The listing builds one solid part. Answer for the finished solid, in the listing's coordinates (mm). Face numbers are marked on the shaded views. Round coordinates to 2 decimals unless told otherwise and drop trailing zeros. Order: outer loops, then holes, each group sorted by start corner. A loop starts at its lowest first (then second) coordinate and runs counter-clockwise, first axis right, second up. Notation, with made-up numbers: (-22.5, 52) -> (-1.5, 52) arc R22 ccw to (-1.5, 78) -> close; hole circle Ø10 at (-11, 1). An arc over 180 degrees is marked (long way). Return JSON: item names as keys, results as strings. Group by question number.
(1) Consider line 1 (Y direction, x = 0, z = 4.4) (3 decimals); line 2 (X direction, y = 0.75, z = 3.7); line 3 (X direction, y = 0.25, z = 0.9). Determine where each line is inside the solid, lowest interval first. Write a range as [from, to].
(2) The part is cut by section D-D (y = 5.75). Determine the outline of the cut face in (x, z).
(3) Determine the mould class of the marked faces 1, 2 and 3 for opening direction Y: +Y half, -Y half, draft (parallel to the pull), parting line (faces both ways), or undercut.
(4) The part is cut by section A-A (z = 3.8). Determine the outline of the cut face in (x, y) (3 decimals).
(5) Each of these flat-tipped pins is pushed along its axis until it touches: pin 1 (2 mm diameter, centred on y = 2.5, z = 3.5, fed in from -X); pin 2 (1 mm diameter, centred on x = -3.5, z = 2.5, fed in from -Y). Where does it stop, or does it pass through?
(6) The part is cut by section C-C (x = -3.25). Determine the outline of the cut face in (y, z), plus the area to 3 significant figures.
(7) The part is cut by section B-B (y = -1). Determine the outline of the cut face in (x, z).
from build123d import *

# Parameters (mm, degrees)
F1_DEPTH = 6


# Not quite as in the source:
# - a feature names something its author has since deleted; it is built from what else it names


with BuildPart() as f1:
    # F0 (on Top) → F1 (new body)
    with BuildSketch(Plane.XY):
        with BuildLine():
            ThreePointArc((0, -7), (4.9497474683, -4.9497474683), (7, 0))
            ThreePointArc((7, 0), (-4.9497474683, 4.9497474683), (0, -7))
        make_face()
        with BuildLine():
            ThreePointArc((3, 2.8311879132), (3.8334465563, 1.5232572009), (4.125, 0))
            ThreePointArc((4.125, 0), (-1.5232572009, -3.8334465563), (-3, 2.8311879132))
            ThreePointArc((-3, 2.8311879132), (0, 4.125), (3, 2.8311879132))
        make_face(mode=Mode.SUBTRACT)
        with BuildLine():
            Line((-3, 2.8311879132), (3, 2.8311879132))
            ThreePointArc((3, 2.8311879132), (0, 4.125), (-3, 2.8311879132))
        make_face()
        with BuildLine():
            ThreePointArc((7.1414284285, -7), (9.2578151927, -3.7805896177), (10, 0))
            ThreePointArc((10, 0), (9.9484557051, 1.0140163134), (9.7943541832, 2.0175792755))
            Line((9.7943541832, 2.0175792755), (7, 0))
            ThreePointArc((7, 0), (4.9497474683, -4.9497474683), (0, -7))
            Line((0, -7), (7.1414284285, -7))
        make_face()
    extrude(amount=F1_DEPTH)


solid = f1.part
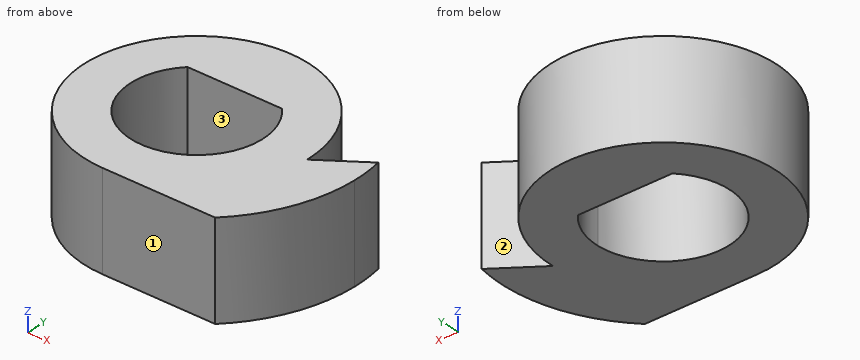
Answer below:
{
 "1": {"line 1": "y = [-7, -4.125], [2.831, 7]", "line 2": "x = [-6.96, -4.06], [4.06, 6.96], [8.04, 9.97]", "line 3": "x = [-7, -4.12], [4.12, 7], [7.35, 10]"},
 "2": {"outline": "(-3.99, 0) -> (3.99, 0) -> (3.99, 6) -> (-3.99, 6) -> close"},
 "3": {"face 1": "-Y half", "face 2": "+Y half", "face 3": "undercut"},
 "4": {"outline": "(0, -7) -> (7.141, -7) arc R10 ccw to (9.794, 2.018) -> (7, 0) arc R7 ccw (long way) to start; hole (-3, 2.831) arc R4.125 ccw (long way) to (3, 2.831) -> close"},
 "5": {"pin 1": "stops at x = -6.84", "pin 2": "stops at y = -6.32"},
 "6": {"outline": "(-6.2, 0) -> (-2.54, 0) -> (-2.54, 6) -> (-6.2, 6) -> close; (2.54, 0) -> (6.2, 0) -> (6.2, 6) -> (2.54, 6) -> close", "area": "43.9 mm²"},
 "7": {"outline": "(-6.93, 0) -> (-4, 0) -> (-4, 6) -> (-6.93, 6) -> close; (4, 0) -> (9.95, 0) -> (9.95, 6) -> (4, 6) -> close"}
}
